```python
from build123d import *

# Parameters (mm, degrees)
F0_W     = 32
F0_H     = 12
F0_R     = 3.25
F1_DEPTH = 2.5
F2_R     = 3
F3_R     = 1


with BuildPart() as f1:
    # F0 (on Top) → F1 (new body)
    with BuildSketch(Plane.XY):
        Rectangle(F0_W, F0_H)
        Circle(F0_R, mode=Mode.SUBTRACT)
    extrude(amount=F1_DEPTH)

    # F2
    f2_edges = [f1.edges().sort_by_distance(p)[0] for p in [
        (-16, 6, 1.25),
        (-16, -6, 1.25),
        (16, 6, 1.25),
        (16, -6, 1.25),
    ]]
    fillet(f2_edges, radius=F2_R)

    # F3
    f3_edges = [f1.edges().sort_by_distance(p)[0] for p in [
        (-3.25, 0, 2.5),
        (-3.25, 0, 0),
    ]]
    fillet(f3_edges, radius=F3_R)


solid = f1.part
```
Source: CAD feature listing. Evaluate the final solid. Frame: model axes, mm. Round coordinates to 2 decimals unless told otherwise and drop trailing zeros. Loops run counter-clockwise (first coordinate to the right, second up) from the corner with the lowest first, then second, coordinate; pieces in that order, holes last. Notation, with made-up numbers: M 76,24 L 119,24 A12 cw 119,47 Z; hole C 59.25,3 d1. An arc over 180 degrees is marked long. Put each result on its own line as item: value.
(1) Section B-B, the plane x = 0. Return loops of the section in (y, z).
Solutions:
outline: M -6,0 L -4.25,0 A1 ccw -3.25,1 L -3.25,1.5 A1 ccw -4.25,2.5 L -6,2.5 Z; M 3.25,1 A1 ccw 4.25,0 L 6,0 L 6,2.5 L 4.25,2.5 A1 ccw 3.25,1.5 Z
(2) Section C-C, the plane z = 0.6. Return loops of the section in (x, y).
Solutions:
outline: M -16,-3 A3 ccw -13,-6 L 13,-6 A3 ccw 16,-3 L 16,3 A3 ccw 13,6 L -13,6 A3 ccw -16,3 Z; hole C 0,0 d6.67
(3) First-contact query: pin 1 (2 mm diameter, centred on x = 1, y = -2.5, fed in from +Z). Flat tip, straight axial feed; report the tip coordinate or a pass-through.
Solutions:
pin 1: z = 2.33
(4) Section A-A, the plane y = 0. Return loops of the section in (x, z), and give its area (3 significant figures).
Solutions:
outline: M -16,0 L -4.25,0 A1 ccw -3.25,1 L -3.25,1.5 A1 ccw -4.25,2.5 L -16,2.5 Z; M 3.25,1 A1 ccw 4.25,0 L 16,0 L 16,2.5 L 4.25,2.5 A1 ccw 3.25,1.5 Z
area: 62.9 mm²
(5) Pull-direction query (X, two-part tool) for faces 1 (the face through (0, -6, 1)), 2 (the face through (-15.14, -5.1, 1.27)), 3 (the face through (15.1, -5.14, 1.27)), 4 (the face through (-2.579, -1.978, 1.246)); classes: released by +X, released by -X, zero draft, split by the parting line, or undercut.
Solutions:
face 1: zero draft
face 2: released by -X
face 3: released by +X
face 4: undercut
(6) Ray query, line 1 (Y direction, x = 0, z = 1.2); line 2 (X direction, y = -3, z = 0.45); line 3 (Y direction, x = -1, z = 0.8). Return the intervals inside material, ascending. Write a range as [from, to].
Solutions:
line 1: [-6, -3.25], [3.25, 6]
line 2: [-16, -1.63], [1.63, 16]
line 3: [-6, -3.11], [3.11, 6]
